from build123d import *

# Parameters (mm, degrees)
F0_W     = 115
F0_H     = 88
F1_DEPTH = 40
F2_T     = -2.5
F3_W     = 15
F3_H     = 5
F3_W_2   = 14
F3_H_2   = 11
F3_W_3   = 11
F3_H_3   = 13
F4_DEPTH = 2.5
F5_R     = 3


with BuildPart() as f1:
    # F0 (on Top) → F1 (new body)
    with BuildSketch(Plane.XY):
        with Locations((2.412276, -2.127609)):
            Rectangle(F0_W, F0_H)
    extrude(amount=F1_DEPTH)

    # F2
    f2_openings = [f1.faces().sort_by_distance(p)[0] for p in [
        (2.412276, -2.127609, 40),
    ]]
    offset(amount=F2_T, openings=f2_openings)

    # F3 (on face) → F4 (cut)
    with BuildSketch(Plane(origin=(0, 41.872391, 0), x_dir=(-1, 0, 0), z_dir=(0, 1, 0))):
        with Locations((7.879983, 31.778646)):
            Rectangle(F3_W, F3_H)
        with Locations((4.874999, 20.622397)):
            Rectangle(F3_W_2, F3_H_2)
        with Locations((42.508882, 13.5)):
            Rectangle(F3_W_3, F3_H_3)
    extrude(amount=-F4_DEPTH, mode=Mode.SUBTRACT)

    # F5
    f5_edges = [f1.edges().sort_by_distance(p)[0] for p in [
        (59.912276, -46.127609, 20),
        (-55.087724, -46.127609, 20),
        (-55.087724, 41.872391, 20),
        (59.912276, 41.872391, 20),
    ]]
    fillet(f5_edges, radius=F5_R)


solid = f1.part
Work out the finished part from the listing and answer in its coordinate system (mm). A direction names the side the tool comes from. Coordinates: 2 decimals unless noted, no trailing zeros. Write each loop counter-clockwise with the first axis right and the second up, starting at its lowest first coordinate (ties: lowest second). Pieces come first, ordered by that corner, then holes. Notation, with made-up numbers: M 4,-11.5 L 17,-11.5 A33 ccw 17,23.5 Z; hole C 34.5,52 d2. An arc over 180 degrees is marked long. Answer as CSV lines item,"result". Start each with the question number.
Item 1: Section D-D on x = 40 is taken. Write down the section's boundary in (y, z).
Item 2: Consider L1, parallel to X at y = 16, z = 20; L2, parallel to Y at x = 18, z = 20; L3, parallel to Z at x = 0, y = -27. Determine where each line is inside the solid, lowest interval first.
Item 3: Flat-ended cylindrical pins translate along their axes: P1, Ø0.8, axis at y = 40, z = 31, coming from the -X side; P2, Ø3, axis at x = -45, y = 41, coming from the -Z side; P3, Ø5, axis at x = -38.5, y = 20.5, coming from the +Z side; P4, Ø1.2, axis at y = 41, z = 14, coming from the +X side. Find the tip coordinate at first contact, or state that the pin passes through.
Item 4: Section A-A on x = -10.5 is taken. Write down the section's boundary in (y, z).
Item 5: Section B-B on z = 16.5 is taken. Write down the section's boundary in (x, y) (3 decimals), and give its area (3 significant figures).
Item 6: A tool of negligible diameter and unlimited length cuts with its end or side. For faces 1 (the face through (-52.588, -3, 21)), 2 (the face through (2, 41.872, 29)), 3 (the face through (-8, 41, 34.279)), from which of +Z, -Z, +X, -X, +Y, -Y can it reach the whole face along a straight path? Write none if from no direction.
Item 7: Determine the mould class of faces 4 (the face through (-42, 41, 7)), 5 (the face through (-54.2, 41, 20.3)), 6 (the face through (59.912, -3, 20)) for opening direction X: released by +X, released by -X, zero draft, split by the parting line, or undercut.
Item 8: Section C-C on y = -8 is taken. Write down the section's boundary in (x, z), and give its area (3 significant figures).
Checks:
1,outline,"M -46.13,0 L 41.87,0 L 41.87,40 L 39.37,40 L 39.37,2.5 L -43.63,2.5 L -43.63,40 L -46.13,40 Z"
2,L1,"x = -55.09 to -52.59, 57.41 to 59.91"
2,L2,"y = -46.13 to -43.63, 39.37 to 41.87"
2,L3,"z = 0 to 2.5"
3,P1,"stops at x = -55"
3,P2,"stops at z = 0"
3,P3,"stops at z = 2.5"
3,P4,"stops at x = 59.49"
4,outline,"M -46.13,0 L 41.87,0 L 41.87,15.12 L 39.37,15.12 L 39.37,2.5 L -43.63,2.5 L -43.63,40 L -46.13,40 Z; M 39.37,26.12 L 41.87,26.12 L 41.87,29.28 L 39.37,29.28 Z; M 39.37,34.28 L 41.87,34.28 L 41.87,40 L 39.37,40 Z"
5,outline,"M -55.088,-43.128 A3 ccw -52.088,-46.128 L 56.912,-46.128 A3 ccw 59.912,-43.128 L 59.912,38.872 A3 ccw 56.912,41.872 L 2.125,41.872 L 2.125,39.372 L 57.412,39.372 L 57.412,-43.628 L -52.588,-43.628 L -52.588,39.372 L -48.009,39.372 L -48.009,41.872 L -52.088,41.872 A3 ccw -55.088,38.872 Z; M -37.009,39.372 L -11.875,39.372 L -11.875,41.872 L -37.009,41.872 Z"
5,area,"920 mm²"
6,face 1,"+Z"
6,face 2,"+Z, -Z, +X, -X, +Y"
6,face 3,"+Y"
7,face 4,"undercut"
7,face 5,"released by -X"
7,face 6,"released by +X"
8,outline,"M -55.09,0 L 59.91,0 L 59.91,40 L 57.41,40 L 57.41,2.5 L -52.59,2.5 L -52.59,40 L -55.09,40 Z"
8,area,"475 mm²"
